Work out the finished part from the listing and answer in its coordinate system (mm). A direction names the side the tool comes from. Round coordinates to 2 decimals unless told otherwise and drop trailing zeros. Write each loop counter-clockwise with the first axis right and the second up, starting at its lowest first coordinate (ties: lowest second). Pieces come first, ordered by that corner, then holes. Notation, with made-up numbers: (-40, -38) -> (-7, -38) arc R17 cw to (-7, -19) -> close; hole circle Ø6 at (53.25, 3). An arc over 180 degrees is marked (long way). One line per item, written item: value.
```python
from build123d import *

# Parameters (mm, degrees)
SKETCH1_W           = 225
SKETCH1_H           = 20
BOSS_EXTRUDE1_DEPTH = 5
SKETCH2_R           = 2.5
BOSS_EXTRUDE2_DEPTH = 15
SKETCH3_R           = 2.5
BOSS_EXTRUDE3_DEPTH = 15
SKETCH4_W           = 215
SKETCH4_H           = 10
CUT_EXTRUDE1_DEPTH  = 6


with BuildPart() as part:
    # Sketch1 → Boss-Extrude1 (new body)
    with BuildSketch(Plane.XY):
        with Locations((112.5, 10)):
            Rectangle(SKETCH1_W, SKETCH1_H)
    extrude(amount=BOSS_EXTRUDE1_DEPTH)

    # Sketch2 → Boss-Extrude2 (add)
    with BuildSketch(Plane(origin=(225, 0, 0), x_dir=(0, 0, -1), z_dir=(1, 0, 0))):
        with Locations((-2.5, 10)):
            Circle(SKETCH2_R)
    extrude(amount=BOSS_EXTRUDE2_DEPTH)

    # Sketch3 → Boss-Extrude3 (add)
    with BuildSketch(Plane.ZY):
        with Locations((2.5, 10)):
            Circle(SKETCH3_R)
    extrude(amount=BOSS_EXTRUDE3_DEPTH)

    # Sketch4 → Cut-Extrude1 (cut, through all)
    with BuildSketch(Plane.XY.offset(5)):
        with Locations((112.5, 10)):
            Rectangle(SKETCH4_W, SKETCH4_H)
    extrude(amount=-CUT_EXTRUDE1_DEPTH, mode=Mode.SUBTRACT)


solid = part.part
```
(1) For a pull along X with two mould halves and no side action, classify faces 1 (the face through (225, 16, 2)), 2 (the face through (111, 5, 3)), 3 (the face through (-7.4, 7.56, 1.96)), 4 (the face through (111, 15, 3)) as pulls with the +X half, pulls with the -X half, needs draft (parallel to the pull), parting line crosses it, or undercut.
Reported:
face 1: pulls with the +X half
face 2: undercut
face 3: needs draft
face 4: undercut
(2) A tool of negligible diameter and unlimited length cuts with its end or side. For faces 5 (the face through (5, 10, 3)), 6 (the face through (111, 17, 0)), 7 (the face through (232.4, 7.56, 3.04)), from which of +Z, -Z, +X, -X, +Y, -Y can it reach the whole face along a straight path? Write none if from no direction.
Reported:
face 5: +Z, -Z
face 6: -Z, +X, -X, +Y, -Y
face 7: +X
(3) Flat-ended cylindrical pins translate along their axes: pin 1 Ø2.5 at (y, z) = (14, 3.5) entering from +X; pin 2 Ø2 at (y, z) = (17.5, 2.5) entering from -X. Find the tip coordinate at first contact, or state that the pin passes through.
Reported:
pin 1: stops at x = 225
pin 2: stops at x = 0
(4) Find section B-B on z = 2.5. Give the vertices of the cut face in (x, y).
Reported:
outline: (-15, 7.5) -> (0, 7.5) -> (0, 0) -> (225, 0) -> (225, 7.5) -> (240, 7.5) -> (240, 12.5) -> (225, 12.5) -> (225, 20) -> (0, 20) -> (0, 12.5) -> (-15, 12.5) -> close; hole (5, 5) -> (220, 5) -> (220, 15) -> (5, 15) -> close
(5) Consider probe 1 along Y at (x, z) = (177.5, 0.9); probe 2 along X at (y, z) = (9.75, 3.05); probe 3 along X at (y, z) = (14.5, 2.4). Determine where each line is inside the solid, lowest interval first.
Reported:
probe 1: y = 0 to 5, 15 to 20
probe 2: x = -15 to 5, 220 to 240
probe 3: x = 0 to 5, 220 to 225
(6) Find section A-A on x = 128. Give the vertices of the cut face in (y, z), plus the area to 3 significant figures.
Reported:
outline: (0, 0) -> (5, 0) -> (5, 5) -> (0, 5) -> close; (15, 0) -> (20, 0) -> (20, 5) -> (15, 5) -> close
area: 50.0 mm2
